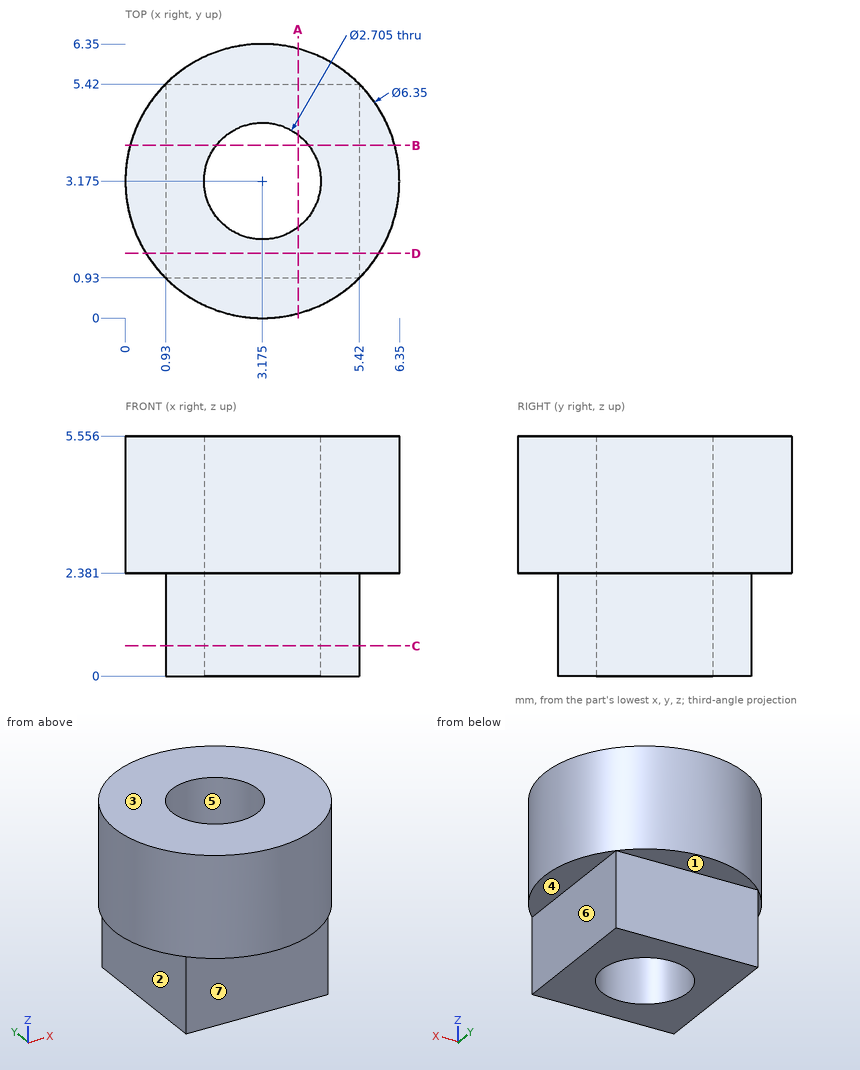
Here's the drawing with two shaded views (mm, measured from the low corner). I have some questions. A direction names the side the tool comes from. Round coordinates to 2 decimals unless told otherwise and drop trailing zeros. Write each loop counter-clockwise with the first axis right and the second up, starting at its lowest first coordinate (ties: lowest second). Pieces come first, ordered by that corner, then holes. Notation, with made-up numbers: M 54.5,-37 L 96.5,-37 A20 ccw 96.5,-30 Z; hole C 8.5,-27.5 d2. An arc over 180 degrees is marked long. Write each question's results on one line, items separated by ' | '. Start each with the question number.
1. On a 3-axis mill with a long thin cutter (end or side, diameter ignored), from which of +Z, -Z, +X, -X, +Y, -Y can I reach the whole of each face in a straight line? I mean the marked faces 1, 2, 3 and 4. Say none if no direction works.
2. Imagine slicing it at A-A on x = 4. List the corners of the cut face in (y, z) for me.
3. I'm going to push flat-ended pins straight in: pin 1 Ø3.5 at (x, y) = (3.175, 3.175) entering from -Z; pin 2 Ø0.7 at (x, z) = (4.5, 1.5) entering from -Y; pin 3 Ø0.7 at (y, z) = (3, 1.5) entering from +X; pin 4 Ø1.2 at (y, z) = (3.5, 1.5) entering from -X. Where does each tip first touch, or does it pass through?
4. Thinking about a two-plate mould opening in X: for the marked faces 5, 6 and 7, which applies, +X half, -X half, draft (parallel to the pull), parting line (faces both ways), or undercut?
5. I need wall thicknesses on L1, parallel to Z at x = 6, y = 2.75; L2, parallel to X at y = 2.75, z = 3.7; L3, parallel to X at y = 2, z = 0.95 (1 decimal). Which ranges of each line are inside material? Lowest first, please. Write a range as from..to.
6. Imagine slicing it at C-C on z = 0.7. List the corners of the cut face in (x, y) for me (1 decimal).
7. Imagine slicing it at D-D on y = 1.5. List the corners of the cut face in (x, z) for me.
Result sheet:
1) face 1: -Z, +X, -X, +Y | face 2: -Z, -X, +Y, -Y | face 3: +Z, +X, -X, +Y, -Y | face 4: -Z, +X, +Y, -Y
2) outline: M 0.11,2.38 L 0.93,2.38 L 0.93,0 L 2.1,0 L 2.1,5.56 L 0.11,5.56 Z; M 4.25,0 L 5.42,0 L 5.42,2.38 L 6.24,2.38 L 6.24,5.56 L 4.25,5.56 Z
3) pin 1: stops at z = 0 | pin 2: stops at y = 0.93 | pin 3: stops at x = 5.42 | pin 4: stops at x = 0.93
4) face 5: undercut | face 6: +X half | face 7: draft
5) L1: z = 2.38..5.56 | L2: x = 0.03..1.89, 4.46..6.32 | L3: x = 0.9..2.5, 3.8..5.4
6) outline: M 0.9,0.9 L 5.4,0.9 L 5.4,5.4 L 0.9,5.4 Z; hole C 3.2,3.2 d2.7
7) outline: M 0.48,2.38 L 0.93,2.38 L 0.93,0 L 5.42,0 L 5.42,2.38 L 5.87,2.38 L 5.87,5.56 L 0.48,5.56 Z
